from build123d import *

# Parameters (mm, degrees)
F0_W      = 4.7
F0_H      = 2.4
F1_DEPTH  = 12.6
F3_DEPTH  = 4.2
F4_R      = 2.3
F4_R_2    = 0.9
F5_DEPTH  = 2.5
F7_DEPTH  = 25
F8_R      = 0.5
F9_W      = 3.8
F9_H      = 1.5
F10_DEPTH = 1


with BuildPart() as f1:
    # F0 (on Front) → F1 (new body)
    with BuildSketch(Plane.XZ):
        Polygon((0, 15.8), (0, 0), (23, 0), (23, 15.8), (23, 18.2), (23, 22.5), (0, 22.5), (0, 18.2), align=None)
        with Locations((-2.35, 17)):
            Rectangle(F0_W, F0_H)
        with Locations((25.35, 17)):
            Rectangle(F0_W, F0_H)
    extrude(amount=F1_DEPTH)

    # F2 (on face) → F3 (join)
    with BuildSketch(Plane.XY.offset(22.5)):
        with BuildLine():
            ThreePointArc((10.916667, -3.801389), (8.5, -6.3), (10.916667, -8.798611))
            ThreePointArc((10.916667, -8.798611), (23, -6.3), (10.916667, -3.801389))
        make_face()
    extrude(amount=F3_DEPTH)

    # F4 (on face) → F5 (join)
    with BuildSketch(Plane.XY.offset(26.7)):
        with Locations((16.7, -6.3)):
            Circle(F4_R)
        with Locations((16.7, -6.3)):
            Circle(F4_R_2, mode=Mode.SUBTRACT)
    extrude(amount=F5_DEPTH)

    # F6 (on face) → F7 (cut)
    with BuildSketch(Plane.XY.offset(18.2)):
        with BuildLine():
            Line((-5.387607, -6.9), (-3.261684, -6.9))
            ThreePointArc((-3.261684, -6.9), (-1.35, -6.3), (-3.261684, -5.7))
            Line((-3.261684, -5.7), (-5.387607, -5.7))
            Line((-5.387607, -5.7), (-5.387607, -6.9))
        make_face()
        with BuildLine():
            ThreePointArc((26.261684, -5.7), (24.35, -6.3), (26.261684, -6.9))
            Line((26.261684, -6.9), (28.387607, -6.9))
            Line((28.387607, -6.9), (28.387607, -5.7))
            Line((28.387607, -5.7), (26.261684, -5.7))
        make_face()
    extrude(amount=-F7_DEPTH, mode=Mode.SUBTRACT)

    # F8
    f8_edges = [f1.edges().sort_by_distance(p)[0] for p in [
        (0, -12.6, 20.35),
        (0, -12.6, 7.9),
        (0, 0, 20.35),
        (0, 0, 7.9),
        (-4.7, -12.6, 17),
        (-4.7, 0, 17),
        (27.7, -12.6, 17),
        (23, -12.6, 20.35),
        (23, -12.6, 7.9),
        (27.7, 0, 17),
        (23, 0, 20.35),
        (23, 0, 7.9),
    ]]
    fillet(f8_edges, radius=F8_R)

    # F9 (on face) → F10 (cut)
    with BuildSketch(Plane.YZ.offset(23)):
        with Locations((-6.3, 4.75)):
            Rectangle(F9_W, F9_H)
    extrude(amount=-F10_DEPTH, mode=Mode.SUBTRACT)


solid = f1.part
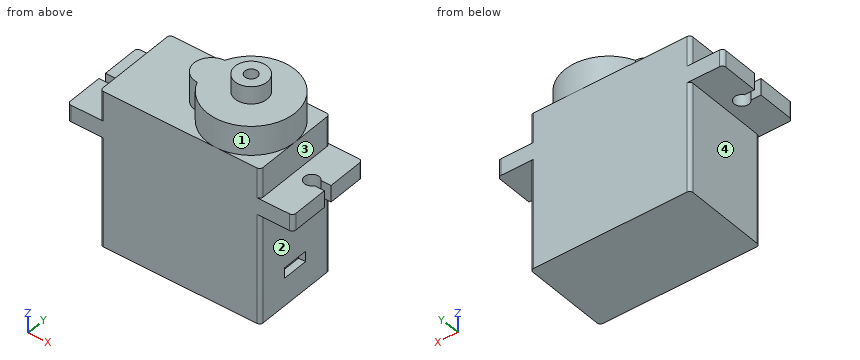
Can you work these out from the model? Positions are in its coordinate system, mm. Face numbers are marked on the shaded views. A direction names the side the tool comes from. Round coordinates to 2 decimals unless told otherwise and drop trailing zeros. Write each loop counter-clockwise with the first axis right and the second up, starting at its lowest first coordinate (ties: lowest second). Pieces come first, ordered by that corner, then holes. Notation, with made-up numbers: (-29.5, 88.5) - (16.5, 88.5) arc R21 ccw to (16.5, 115.5) - close; hole circle Ø11 at (87.5, 33.5). An arc over 180 degrees is marked (long way). Write each question's results on one line, items separated by ' | '. Start each with the question number.
1) Suppose I cut it at C-C (y = -11.25). List the corners of the cut face in (x, z) for me, and give its area (3 significant figures).
2) Which directions (+Z, -Z, +X, -X, +Y, -Y) give clear straight access to the entire face, cutting with the end or side of a thin tool? Please do the marked faces 1, 2, 3 and 4.
3) Suppose I cut it at D-D (x = 7.5). List the corners of the cut face in (y, z) for me, and give its area (4 significant figures).
4) Suppose I cut it at A-A (x = -2.4). List the corners of the cut face in (y, z) for me, and give its area (3 significant figures).
5) Please list where these lines run through material, in increasing order: line 1 (Y direction, x = -2.4, z = 17); line 2 (X direction, y = -7, z = 22); line 3 (Z direction, x = 14, y = -8.5).
6) Suppose I cut it at B-B (z = 10.75). List the corners of the cut face in (x, y) for me.
7) For pin 1 Ø5 at (x, z) = (0, 8.5) entering from -Y; pin 2 Ø5 at (x, y) = (10.5, -4) entering from +Z; pin 3 Ø3.5 at (x, y) = (-2.4, -6.3) entering from -Z; pin 4 Ø1.6 at (x, y) = (26, -6.5) entering from +Z, each with a flat end and sliding along its axis, tell me the tip position at first contact or that it passes through.
Here are the results:
1) outline: (-4.7, 15.8) - (0, 15.8) - (0, 0) - (23, 0) - (23, 15.8) - (27.7, 15.8) - (27.7, 18.2) - (23, 18.2) - (23, 22.5) - (20.6, 22.5) - (20.6, 26.7) - (12.8, 26.7) - (12.8, 22.5) - (0, 22.5) - (0, 18.2) - (-4.7, 18.2) - close | area: 573 mm2
2) face 1: +Z | face 2: -Z, +X, +Y, -Y | face 3: +Z, +X, +Y, -Y | face 4: -Z, -X, +Y, -Y
3) outline: (-12.6, 0) - (0, 0) - (0, 22.5) - (-12.6, 22.5) - close | area: 283.5 mm2
4) outline: (-12.6, 15.8) - (-7.35, 15.8) - (-7.35, 18.2) - (-12.6, 18.2) - close; (-5.25, 15.8) - (0, 15.8) - (0, 18.2) - (-5.25, 18.2) - close | area: 25.2 mm2
5) line 1: y = -12.6 to -7.35, -5.25 to 0 | line 2: x = 0 to 23 | line 3: z = 0 to 26.7
6) outline: (0, -12.1) arc R0.5 ccw to (0.5, -12.6) - (22.5, -12.6) arc R0.5 ccw to (23, -12.1) - (23, -0.5) arc R0.5 ccw to (22.5, 0) - (0.5, 0) arc R0.5 ccw to (0, -0.5) - close
7) pin 1: stops at y = -12.6 | pin 2: stops at z = 26.7 | pin 3: stops at z = 15.8 | pin 4: stops at z = 18.2
